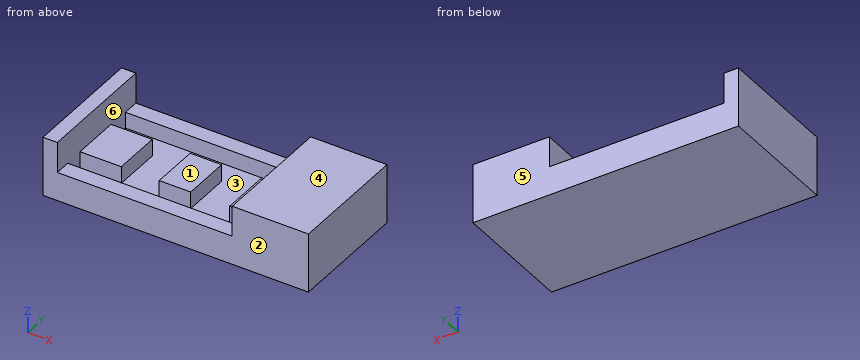
```python
from build123d import *

# Parameters (mm, degrees)
F0_W     = 192.0494
F0_H     = 88.4428
F1_DEPTH = 42.926
F2_W     = 126.5174
F2_H     = 88.4428
F3_DEPTH = 22.1488
F4_W     = 126.5174
F4_H     = 64.9732
F5_DEPTH = 11.7348
F6_W     = 29.845
F6_H     = 34.8996
F6_W_2   = 22.7584
F6_W_3   = 18.2626
F7_DEPTH = 12.2428


with BuildPart() as f1:
    # F0 (on Top) → F1 (new body)
    with BuildSketch(Plane.XY):
        with Locations((96.0247, 44.2214)):
            Rectangle(F0_W, F0_H)
    extrude(amount=F1_DEPTH)

    # F2 (on face) → F3 (cut)
    with BuildSketch(Plane.XY.offset(42.926)):
        with Locations((73.6219, 44.2214)):
            Rectangle(F2_W, F2_H)
    extrude(amount=-F3_DEPTH, mode=Mode.SUBTRACT)

    # F4 (on face) → F5 (cut)
    with BuildSketch(Plane.XY.offset(20.7772)):
        with Locations((73.6219, 44.2214)):
            Rectangle(F4_W, F4_H)
    extrude(amount=-F5_DEPTH, mode=Mode.SUBTRACT)

    # F6 (on face) → F7 (join)
    with BuildSketch(Plane.XY.offset(9.0424)):
        with Locations((25.2857, 43.0276)):
            Rectangle(F6_W, F6_H)
        with Locations((79.0448, 43.0276)):
            Rectangle(F6_W_2, F6_H)
        with Locations((127.7493, 43.0276)):
            Rectangle(F6_W_3, F6_H)
    extrude(amount=F7_DEPTH)


solid = f1.part
```
The model under review builds one solid part; all positions refer to its coordinate system, in mm. Face numbers are marked on the shaded views. A direction names the side the tool comes from. Coordinates: 2 decimals unless noted, no trailing zeros. Write each loop counter-clockwise with the first axis right and the second up, starting at its lowest first coordinate (ties: lowest second). Pieces come first, ordered by that corner, then holes. Notation, with made-up numbers: (-32, 30.5) - (21, 30.5) arc R26 cw to (21, 56.5) - close; hole circle Ø10 at (56.5, -21.75). An arc over 180 degrees is marked (long way). Answer in a Markdown table with one row per item. Add a question column.
Q1. Consider section B-B on x = 16. Give the boundary of the cut face in (y, z), then the cut area to 3 significant figures.
Q2. Consider section D-D on x = 96.5. Give the boundary of the cut face in (y, z).
Q3. For the marked faces 1 and 2, list the 3-axis set-ups (+Z, -Z, +X, -X, +Y, -Y) from which the entire face can be reached by the end or side of a thin tool; tool diameter is ignored.
Q4. Clearance check with flat-ended pins moving along their axes: pin 1 (13 mm diameter, centred on x = 97.5, y = 82, fed in from +Z); pin 2 (5.5 mm diameter, centred on x = 128, y = 45, fed in from +Z). State where each tip first meets the part, or that it passes through.
Q5. Consider section C-C on y = 62.5. Give the boundary of the cut face in (x, z), then the cut area to 3 significant figures.
Q6. Consider section A-A on z = 30. Give the boundary of the cut face in (x, y), then the cut area to 3 significant figures.
Q7. Draft analysis for pull direction Y (two halves, no side actions). For the marked faces 3, 4, 5 and 6, state which applies: +Y half, -Y half, draft (parallel to the pull), parting line (faces both ways), or undercut.
Q8. To check wall thickness, follow line 1 along X through (y, z) = (42, 19.5); line 2 along Y through (x, z) = (88.5, 12.5); line 3 along X through (y, z) = (38, 41.5). State the ranges of each line that lie inside material, in increasing order. Write a range as from..to.
Answers below:
| question | item | result |
|---|---|---|
| 1 | outline | (0, 0) - (88.44, 0) - (88.44, 20.78) - (76.71, 20.78) - (76.71, 9.04) - (60.48, 9.04) - (60.48, 21.29) - (25.58, 21.29) - (25.58, 9.04) - (11.73, 9.04) - (11.73, 20.78) - (0, 20.78) - close |
| 1 | area | 1,500 mm² |
| 2 | outline | (0, 0) - (88.44, 0) - (88.44, 20.78) - (76.71, 20.78) - (76.71, 9.04) - (11.73, 9.04) - (11.73, 20.78) - (0, 20.78) - close |
| 3 | face 1 | +Z, +Y, -Y |
| 3 | face 2 | +Z, -Z, +X, -X, -Y |
| 4 | pin 1 | z = 20.78 |
| 4 | pin 2 | z = 21.29 |
| 5 | outline | (0, 0) - (192.05, 0) - (192.05, 42.93) - (136.88, 42.93) - (136.88, 9.04) - (10.36, 9.04) - (10.36, 42.93) - (0, 42.93) - close |
| 5 | area | 3,960 mm² |
| 6 | outline | (0, 0) - (10.36, 0) - (10.36, 88.44) - (0, 88.44) - close; (136.88, 0) - (192.05, 0) - (192.05, 88.44) - (136.88, 88.44) - close |
| 6 | area | 5,800 mm² |
| 7 | face 3 | undercut |
| 7 | face 4 | draft |
| 7 | face 5 | +Y half |
| 7 | face 6 | undercut |
| 8 | line 1 | 0..40.21, 67.67..90.42, 118.62..192.05 |
| 8 | line 2 | 0..11.73, 25.58..60.48, 76.71..88.44 |
| 8 | line 3 | 0..10.36, 136.88..192.05 |
